Check sheet for the drawn part. Datum: minimum x, y, z corner. Units: mm. Give positions to 0.01 mm unless a question says otherwise; leave off trailing zeros. Loops run counter-clockwise (first coordinate to the right, second up) from the corner with the lowest first, then second, coordinate; pieces in that order, holes last. Notation, with made-up numbers: (-21, -16.5) - (-12, -16.5) arc R13 ccw to (-12, 6.5) - close; hole circle Ø9 at (66.25, 18). An arc over 180 degrees is marked (long way). One line per item, written item: value. Start each with the question number.
1. Sectioned sample at C-C (y = 2.05). Count the separate pieces of the cut face and the enclosed holes in it, plus the area to 3 significant figures.
2. Scan lines: L1, parallel to X at y = 0.6, z = 44; L2, parallel to X at y = 2.75, z = 50; L3, parallel to Z at x = 290, y = 3.7. Record each from-to range of solid material in increasing order. Write a range as [from, to].
3. Sectioned sample at A-A (z = 40). Record the cut outline in (x, y), plus the area to 3 significant figures.
4. Sectioned sample at B-B (x = 385.5). Record the cut outline in (y, z), plus the area to 3 significant figures.
5. Sectioned sample at D-D (x = 245.5). Record the cut outline in (y, z), plus the area to 3 significant figures.
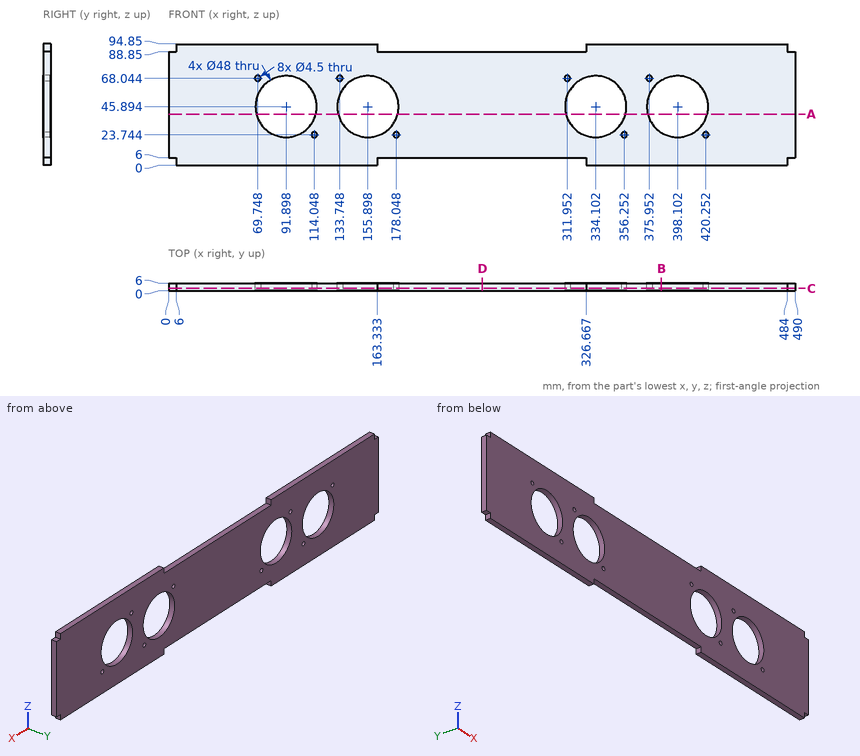
Results are:
1. separate pieces: 1
1. enclosed holes: 12
1. area: 37,000 mm^2
2. L1: x = [0, 67.97], [115.82, 131.97], [179.82, 310.18], [358.03, 374.18], [422.03, 490]
2. L2: x = [0, 68.25], [115.54, 132.25], [179.54, 310.46], [357.75, 374.46], [421.75, 490]
2. L3: z = [6, 88.85]
3. outline: (0, 0) - (68.63, 0) - (68.63, 6) - (0, 6) - close; (115.16, 0) - (132.63, 0) - (132.63, 6) - (115.16, 6) - close; (179.16, 0) - (310.84, 0) - (310.84, 6) - (179.16, 6) - close; (357.37, 0) - (374.84, 0) - (374.84, 6) - (357.37, 6) - close; (421.37, 0) - (490, 0) - (490, 6) - (421.37, 6) - close
3. area: 1,820 mm^2
4. outline: (0, 0) - (6, 0) - (6, 25.47) - (0, 25.47) - close; (0, 66.32) - (6, 66.32) - (6, 94.85) - (0, 94.85) - close
4. area: 324 mm^2
5. outline: (0, 6) - (6, 6) - (6, 88.85) - (0, 88.85) - close
5. area: 497 mm^2
